```python
from build123d import *

# Parameters (mm, degrees)
SKETCH1_W        = 190
SKETCH1_H        = 190
SKETCH1_R        = 37.5
MAIN_PLATE_DEPTH = 3


# Sheet-metal steps are written as plain solids
with BuildPart() as part:
    # Sketch1 → Main Plate (new body)
    with BuildSketch(Plane.XY):
        Rectangle(SKETCH1_W, SKETCH1_H)
        Circle(SKETCH1_R, mode=Mode.SUBTRACT)
    extrude(amount=-MAIN_PLATE_DEPTH)


solid = part.part
```
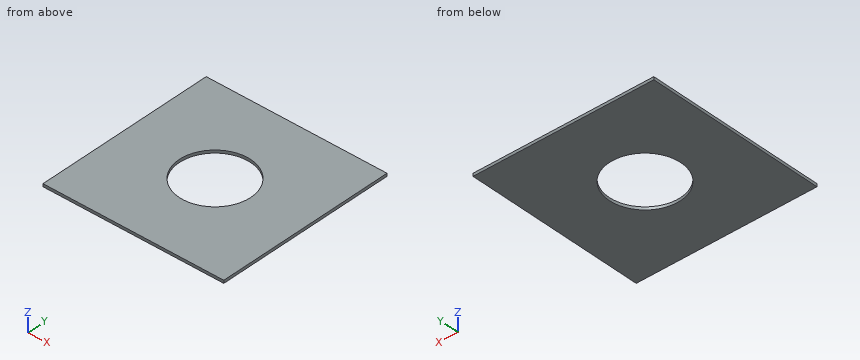
The model under review builds one solid part; all positions refer to its coordinate system, in mm. Round coordinates to 2 decimals unless told otherwise and drop trailing zeros. Loops run counter-clockwise (first coordinate to the right, second up) from the corner with the lowest first, then second, coordinate; pieces in that order, holes last. Notation, with made-up numbers: M 15.5,7 L 34.5,7 A27 cw 34.5,42 Z; hole C 89.5,-8 d7. An arc over 180 degrees is marked long. Put each result on its own line as item: value.
Q1. Consider section A-A, the plane x = 0. Give the boundary of the cut face in (y, z), then the cut area to 3 significant figures.
Result set:
outline: M -95,-3 L -37.5,-3 L -37.5,0 L -95,0 Z; M 37.5,-3 L 95,-3 L 95,0 L 37.5,0 Z
area: 345 mm²
Q2. To check wall thickness, follow L1, parallel to Y at x = 0, z = -1; L2, parallel to Y at x = 3, z = -2.55; L3, parallel to X at y = -26.5, z = -1.65. State the ranges of each line that lie inside material, in increasing order.
Result set:
L1: y = -95 to -37.5, 37.5 to 95
L2: y = -95 to -37.38, 37.38 to 95
L3: x = -95 to -26.53, 26.53 to 95
Q3. Consider section C-C, the plane z = -1.4. Give the boundary of the cut face in (x, y).
Result set:
outline: M -95,-95 L 95,-95 L 95,95 L -95,95 Z; hole C 0,0 d75
